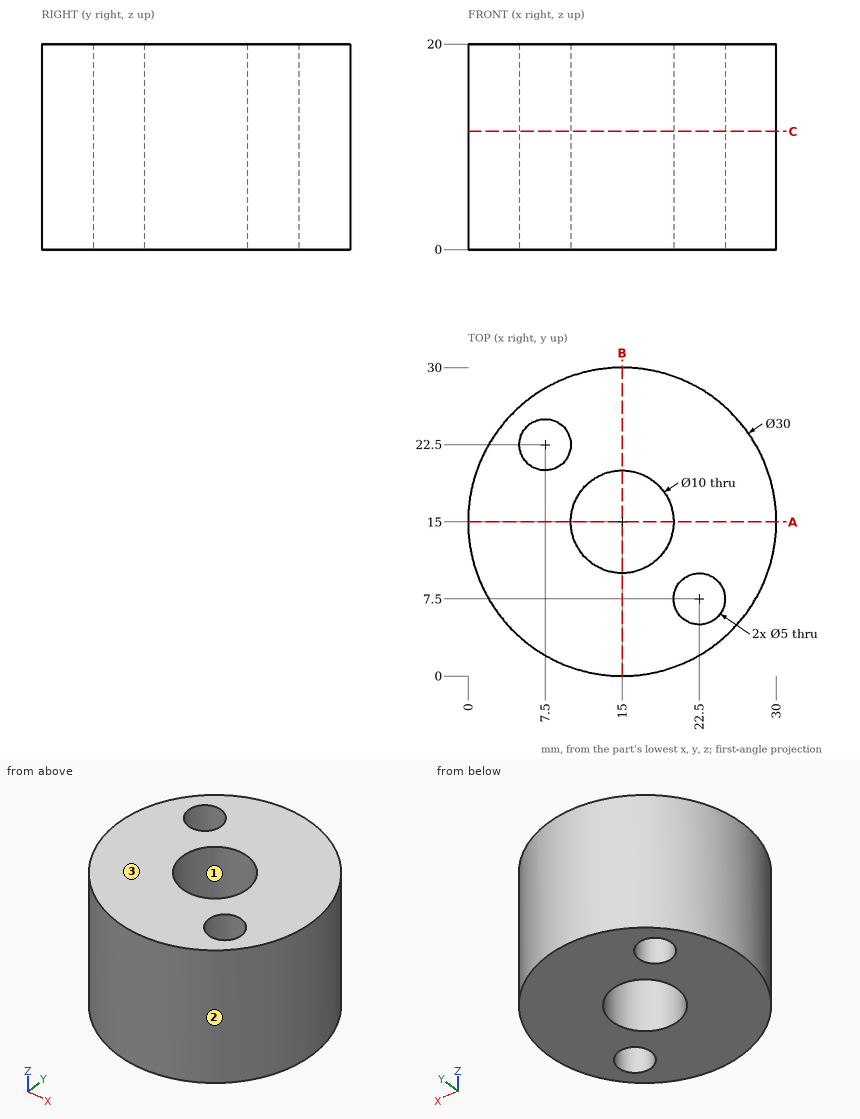
Input: dimensioned drawing with shaded views. Units: mm. Origin: part minimum x, y, z. Give positions to 0.01 mm unless a question says otherwise; leave off trailing zeros. Write each loop counter-clockwise with the first axis right and the second up, starting at its lowest first coordinate (ties: lowest second). Pieces come first, ordered by that corner, then holes.
1. Line query: probe 1 along Y at (x, z) = (15, 9.75); probe 2 along Y at (x, z) = (7.5, 7.75); probe 3 along X at (y, z) = (13.25, 13). Output: solid intervals per line, ascending.
2. Pin query (flat end, axial travel): P1, Ø3, axis at y = 4.5, z = 4, coming from the -X side; P2, Ø6, axis at y = 8.5, z = 9.5, coming from the +X side; P3, Ø4, axis at y = 5.5, z = 13.5, coming from the -X side. Return the tip coordinate at first contact, or that it passes through.
3. Section query A-A, the plane y = 15. Return loops of the section in (x, z), then the cut area to 3 significant figures.
4. Section query C-C, the plane z = 11.5. Return loops of the section in (x, y), then the cut area to 3 significant figures.
5. Draft query along Y for the marked faces 1, 2 and 3. Return one class per face: released by +Y, released by -Y, zero draft, split by the parting line, or undercut.
Computed:
1. probe 1: y = 0 to 10, 20 to 30
1. probe 2: y = 2.01 to 20, 25 to 27.99
1. probe 3: x = 0.1 to 10.32, 19.68 to 29.9
2. P1: stops at x = 3
2. P2: stops at x = 29.59
2. P3: stops at x = 2.01
3. outline: (0, 0) - (10, 0) - (10, 20) - (0, 20) - close; (20, 0) - (30, 0) - (30, 20) - (20, 20) - close
3. area: 400 mm2
4. outline: circle Ø30 at (15, 15); hole circle Ø5 at (7.5, 22.5); hole circle Ø10 at (15, 15); hole circle Ø5 at (22.5, 7.5)
4. area: 589 mm2
5. face 1: undercut
5. face 2: split by the parting line
5. face 3: zero draft
